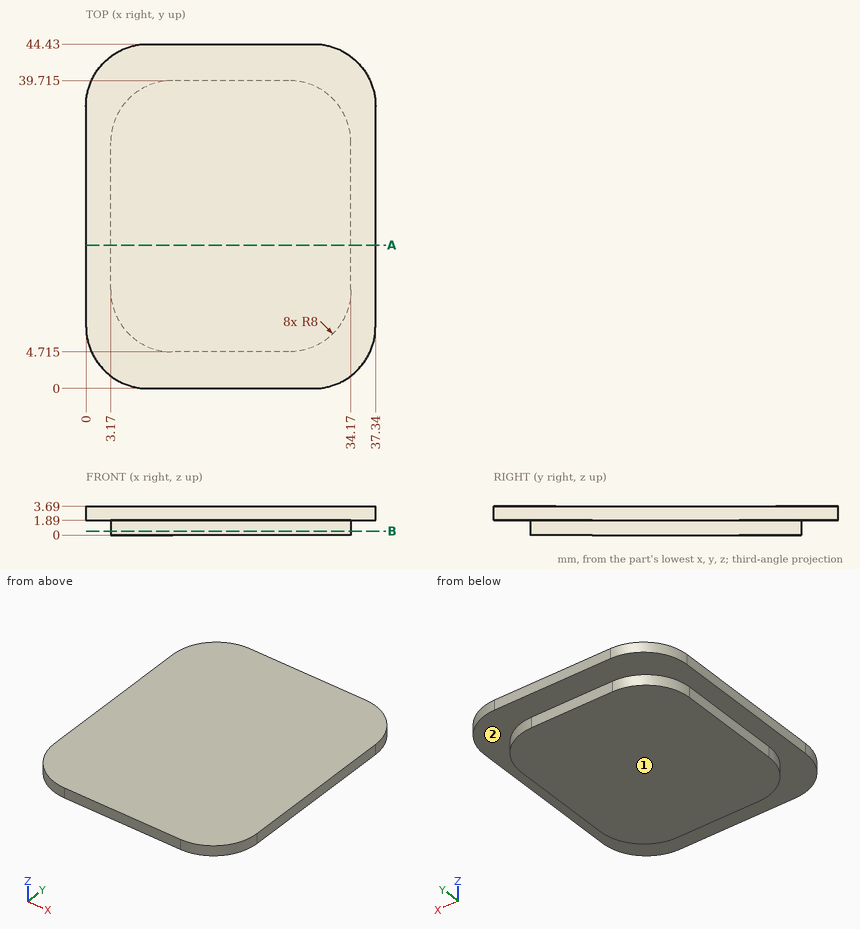
Verification items for this drawing (mm, ordinates from the low corner). A direction names the side the tool comes from. Round coordinates to 2 decimals unless told otherwise and drop trailing zeros. Loops run counter-clockwise (first coordinate to the right, second up) from the corner with the lowest first, then second, coordinate; pieces in that order, holes last. Notation, with made-up numbers: M 41,61 L 51,61 A14 cw 51,75 Z; hole C -20,-21.5 d8. An arc over 180 degrees is marked long. Answer as a JSON object with one key per item and string values.
1. Section check B-B (z = 0.5). Record the boundary of the cut face in (x, y) (3 decimals).
Reply:
{"outline": "M 3.17,12.715 A8 ccw 11.17,4.715 L 26.17,4.715 A8 ccw 34.17,12.715 L 34.17,31.715 A8 ccw 26.17,39.715 L 11.17,39.715 A8 ccw 3.17,31.715 Z"}
2. Scan lines: line 1 (Z direction, x = 36, y = 38); line 2 (X direction, y = 31, z = 0.85); line 3 (Y direction, x = 29.5, z = 1.3). Record each from-to range of solid material in increasing order.
Reply:
{"line 1": "z = 1.89 to 3.69", "line 2": "x = 3.17 to 34.17", "line 3": "y = 5.44 to 38.99"}
3. Access from +Z, -Z, +X, -X, +Y, -Y to the whole of each face (thin tool, end or side, straight path). Record for the marked faces 1 and 2.
Reply:
{"face 1": "-Z, +X, -X, +Y, -Y", "face 2": "-Z"}
4. Gauge pin test, flat ends, axial feed: P1, Ø1.5, axis at x = 21, z = 0.5, coming from the -Y side (3 decimals); P2, Ø0.9, axis at x = 19, z = 1, coming from the +Y side (3 decimals); P3, Ø2, axis at y = 17.5, z = 0.5, coming from the -X side. Record the tip position at first contact, or that the pin passes through.
Reply:
{"P1": "stops at y = 4.715", "P2": "stops at y = 39.715", "P3": "stops at x = 3.17"}
5. Section check A-A (y = 18.5). Record the boundary of the cut face in (x, z), plus the area to 3 significant figures.
Reply:
{"outline": "M 0,1.89 L 3.17,1.89 L 3.17,0 L 34.17,0 L 34.17,1.89 L 37.34,1.89 L 37.34,3.69 L 0,3.69 Z", "area": "126 mm²"}
